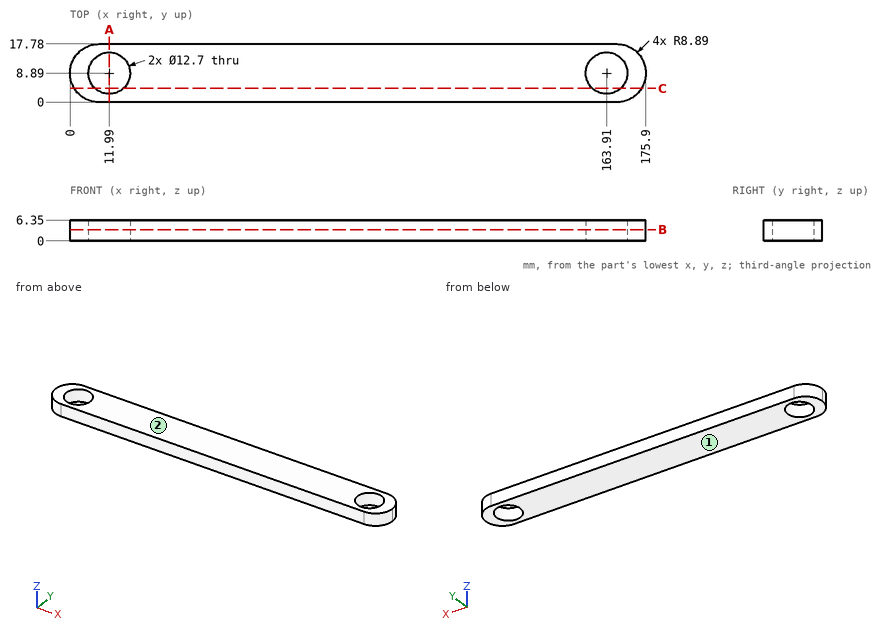
For this review, use the dimensioned drawing (mm, ordinates from the lowest corner) and the shaded views. Give positions to 0.01 mm unless a question says otherwise; leave off trailing zeros. Order: outer loops, then holes, each group sorted by start corner. A loop starts at its lowest first (then second) coordinate and runs counter-clockwise, first axis right, second up. Notation, with made-up numbers: (65, 12) - (123, 12) arc R27 ccw to (123, 36) - close; hole circle Ø7 at (-40, -10.75). An arc over 180 degrees is marked (long way). Use a Markdown table: item, result. Add a question column.
(1) Add section B-B on z = 3.5. Give the number of separate pieces and of enclosed holes in the cut face, then the cut area to 3 significant figures.
(2) Add section A-A on x = 11.99. Give the boundary of the cut face in (y, z), then the cut area to 3 significant figures.
(3) Wall thickness on probe 1 along X at (y, z) = (8.89, 4.25); probe 2 along Y at (x, z) = (163.91, 4.5); probe 3 along X at (y, z) = (5.25, 4): over which ranges is each line inside the solid? List them lowest first. Write a range as [from, to].
(4) Add section C-C on y = 4.25. Give the boundary of the cut face in (x, z) (3 decimals).
(5) Clearance check with flat-ended pins moving along their axes: P1, Ø1.5, axis at y = 13, z = 1.5, coming from the -X side; P2, Ø2, axis at y = 7, z = 1, coming from the +X side; P3, Ø1, axis at y = 15, z = 4, coming from the -X side. State where each tip first meets the part, or that it passes through.
(6) Mouldability with a two-part tool opening along Z and no side actions: class the marked faces 1 and 2 as +Z half, -Z half, draft (parallel to the pull), parting line (faces both ways), or undercut.
Report:
| question | item | result |
|---|---|---|
| 1 | separate pieces | 1 |
| 1 | enclosed holes | 2 |
| 1 | area | 2,810 mm² |
| 2 | outline | (0, 0) - (2.54, 0) - (2.54, 6.35) - (0, 6.35) - close; (15.24, 0) - (17.78, 0) - (17.78, 6.35) - (15.24, 6.35) - close |
| 2 | area | 32.3 mm² |
| 3 | probe 1 | x = [0, 5.64], [18.34, 157.56], [170.26, 175.9] |
| 3 | probe 2 | y = [0, 2.54], [15.24, 17.78] |
| 3 | probe 3 | x = [0.78, 6.79], [17.19, 158.71], [169.11, 175.12] |
| 4 | outline | (1.307, 0) - (7.655, 0) - (7.655, 6.35) - (1.307, 6.35) - close; (16.325, 0) - (159.575, 0) - (159.575, 6.35) - (16.325, 6.35) - close; (168.245, 0) - (174.593, 0) - (174.593, 6.35) - (168.245, 6.35) - close |
| 5 | P1 | stops at x = 0.66 |
| 5 | P2 | stops at x = 175.86 |
| 5 | P3 | stops at x = 1.99 |
| 6 | face 1 | -Z half |
| 6 | face 2 | +Z half |
